Check sheet for the drawn part. Datum: minimum x, y, z corner. Units: mm. Give positions to 0.01 mm unless a question says otherwise; leave off trailing zeros. Write each loop counter-clockwise with the first axis right and the second up, starting at its lowest first coordinate (ties: lowest second). Pieces come first, ordered by that corner, then holes. Notation, with made-up numbers: M 19,-28.75 L 30,-28.75 A28 cw 30,2.25 Z; hole C 72.5,-26.5 d11. An arc over 180 degrees is marked long. Use CSV: the item, a comma, the result in double quotes. Start each with the question number.
1. Cross-section at B-B, the plane y = 127. Enter the section's corners in (x, z), and give its area (3 significant figures).
2. Scan lines: line 1 (Y direction, x = 89, z = 5); line 2 (Y direction, x = 148.9, z = 3.5); line 3 (X direction, y = 210, z = 1.5). Record each from-to range of solid material in increasing order.
3. Cross-section at A-A, the plane x = 28.9. Enter the section's corners in (y, z), and give its area (3 significant figures).
4. Depth check by flat-ended pin: P1, Ø18, axis at x = 28.9, y = 127, coming from the +Z side; P2, Ø10, axis at x = 26.5, y = 224.5, coming from the -Z side. Enter the tip coordinate at first touch or a pass-through.
5. Cross-section at C-C, the plane z = 1.75. State how many separate pieces and enclosed holes the cut face has, and give its area (3 significant figures).
6. Cross-section at D-D, the plane x = 129.5. Enter the section's corners in (y, z).
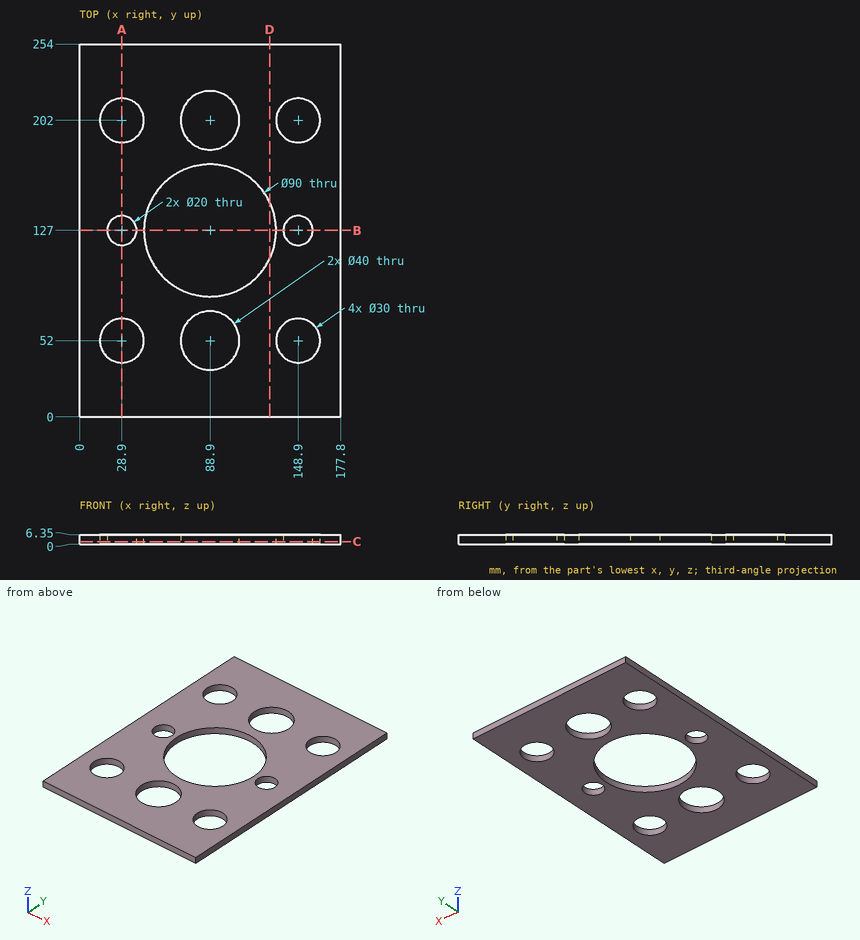
Worked answers:
1,outline,"M 0,0 L 18.9,0 L 18.9,6.35 L 0,6.35 Z; M 38.9,0 L 43.9,0 L 43.9,6.35 L 38.9,6.35 Z; M 133.9,0 L 138.9,0 L 138.9,6.35 L 133.9,6.35 Z; M 158.9,0 L 177.8,0 L 177.8,6.35 L 158.9,6.35 Z"
1,area,"304 mm^2"
2,line 1,"y = 0 to 32, 72 to 82, 172 to 182, 222 to 254"
2,line 2,"y = 0 to 37, 67 to 117, 137 to 187, 217 to 254"
2,line 3,"x = 0 to 16.21, 41.59 to 70.57, 107.23 to 136.21, 161.59 to 177.8"
3,outline,"M 0,0 L 37,0 L 37,6.35 L 0,6.35 Z; M 67,0 L 117,0 L 117,6.35 L 67,6.35 Z; M 137,0 L 187,0 L 187,6.35 L 137,6.35 Z; M 217,0 L 254,0 L 254,6.35 L 217,6.35 Z"
3,area,"1,100 mm^2"
4,P1,"passes through"
4,P2,"stops at z = 0"
5,separate pieces,"1"
5,enclosed holes,"9"
5,area,"32,800 mm^2"
6,outline,"M 0,0 L 107.59,0 L 107.59,6.35 L 0,6.35 Z; M 146.41,0 L 254,0 L 254,6.35 L 146.41,6.35 Z"
